from build123d import *

# Parameters (mm, degrees)
EXTRUDE_1_DEPTH     = 3
FILLET_1_R          = 0.5
CUT_EXTRUDE_1_DEPTH = 2.1


with BuildPart() as part:
    # 草图1 → 凸台-拉伸1 (new body)
    with BuildSketch(Plane(origin=(0, 0, 0), x_dir=(1, 0, 0), z_dir=(0, 1, 0))):
        with BuildLine():
            Line((0, 0), (23.75, 0))
            ThreePointArc((23.75, 0), (30, 6.25), (23.75, 12.5))
            Line((23.75, 12.5), (0, 12.5))
            Line((0, 12.5), (0, 0))
        make_face()
    extrude(amount=EXTRUDE_1_DEPTH)

    # 圆角1
    fillet_1_edges = [part.edges().sort_by_distance(p)[0] for p in [
        (30, 3, -6.25),
        (11.875, 3, -12.5),
        (0, 3, -6.25),
        (11.875, 0, -12.5),
        (30, 0, -6.25),
        (11.875, 0, 0),
        (0, 0, -6.25),
        (0, 1.5, -12.5),
        (0, 1.5, 0),
        (11.875, 3, 0),
    ]]
    fillet(fillet_1_edges, radius=FILLET_1_R)

    # 草图2 → 切除-拉伸1 (cut)
    with BuildSketch(Plane(origin=(0, 3, 0), x_dir=(1, 0, 0), z_dir=(0, 1, 0))):
        with BuildLine():
            Line((9.365836637, 8.148135013), (21.448084588, 8.683862246))
            ThreePointArc((21.448084588, 8.683862246), (27.1, 6.25), (21.448084588, 3.816137754))
            Line((21.448084588, 3.816137754), (9.365836637, 4.351864987))
            ThreePointArc((9.365836637, 4.351864987), (7.55, 6.25), (9.365836637, 8.148135013))
        make_face()
    extrude(amount=-CUT_EXTRUDE_1_DEPTH, mode=Mode.SUBTRACT)


solid = part.part
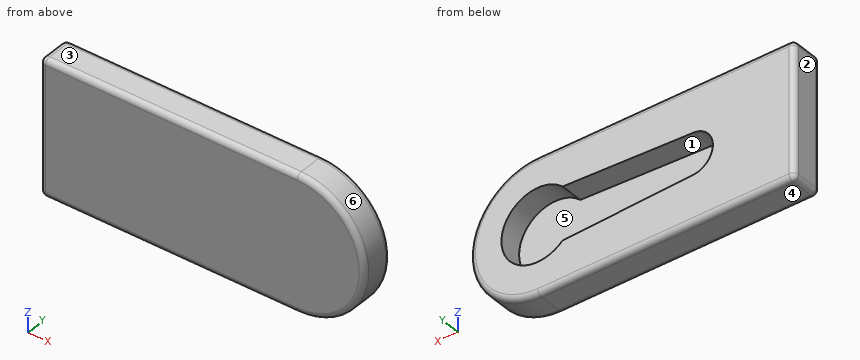
Source: CAD feature listing. Evaluate the final solid. Frame: model axes, mm. Face numbers are marked on the shaded views. A direction names the side the tool comes from. Give positions to 0.01 mm unless a question says otherwise; leave off trailing zeros. Write each loop counter-clockwise with the first axis right and the second up, starting at its lowest first coordinate (ties: lowest second). Pieces come first, ordered by that corner, then holes. Notation, with made-up numbers: (23.5, 68.5) -> (49.5, 68.5) arc R3 cw to (49.5, 73.5) -> close; hole circle Ø9 at (67, 59.25). An arc over 180 degrees is marked (long way). Write item = value, one per line.
Q1. Mould query, pull axis Z, two halves, no side actions, for the marked faces 1, 2, 3 and 4. Classes: +Z half, -Z half, draft (parallel to the pull), parting line (faces both ways), or undercut.
Here are the results:
face_1 = undercut
face_2 = draft
face_3 = +Z half
face_4 = -Z half
Q2. Cut plane C-C on z = -6.25. Return loops of the section in (x, y), then the cut area to 3 significant figures.
Here are the results:
outline = (0, 0.5) arc R0.5 ccw to (0.5, 0) -> (29.5, 0) arc R0.5 ccw to (30, 0.5) -> (30, 2.5) arc R0.5 ccw to (29.5, 3) -> (27.1, 3) -> (27.1, 0.9) -> (7.55, 0.9) -> (7.55, 3) -> (0.5, 3) arc R0.5 ccw to (0, 2.5) -> close
area = 48.7 mm²
Q3. Cut plane B-B on x = 18. Return loops of the section in (y, z).
Here are the results:
outline = (0, -12) arc R0.5 ccw to (0.5, -12.5) -> (2.5, -12.5) arc R0.5 ccw to (3, -12) -> (3, -8.53) -> (0.9, -8.53) -> (0.9, -3.97) -> (3, -3.97) -> (3, -0.5) arc R0.5 ccw to (2.5, 0) -> (0.5, 0) arc R0.5 ccw to (0, -0.5) -> close
Q4. First-contact query: pin 1 (7.5 mm diameter, centred on x = 20, z = -7, fed in from +Y); pin 2 (1 mm diameter, centred on y = 1, z = -7.5, fed in from +X); pin 3 (5.5 mm diameter, centred on x = 23.75, z = -6.25, fed in from +Y). Flat tips, straight axial feed; report the tip coordinate or a pass-through.
Here are the results:
pin_1 = 3
pin_2 = 29.95
pin_3 = 0.9
Q5. Reachability of the marked faces 5 and 6 from +Z, -Z, +X, -X, +Y, -Y: full face, straight path, thin tool, end or side. Return the list, or none.
Here are the results:
face_5 = +Y
face_6 = +X, +Y, -Y
Q6. Line query: line 1 (Z direction, x = 23.75, y = 1.45); line 2 (X direction, y = 2.8, z = -8.75); line 3 (Z direction, x = 19, y = 2.4). Output: solid intervals per line, ascending. Write a range as from..to.
Here are the results:
line_1 = -12.5..-9.6, -2.9..0
line_2 = 0.1..21.52, 25.98..29.37
line_3 = -12.5..-8.58, -3.92..0
Q7. Cut plane A-A on y = 1.2. Return loops of the section in (x, z).
Here are the results:
outline = (0, -12) arc R0.5 ccw to (0.5, -12.5) -> (23.75, -12.5) arc R6.25 ccw to (23.75, 0) -> (0.5, 0) arc R0.5 ccw to (0, -0.5) -> close; hole (9.37, -8.15) -> (21.45, -8.68) arc R3.35 ccw (long way) to (21.45, -3.82) -> (9.37, -4.35) arc R1.9 ccw to start
